```python
from build123d import *

# Parameters (mm, degrees)
F1_DEPTH = 10.4775
F2_R     = 1.5875
F3_DEPTH = 2.54
F4_R     = 0.79375
F5_DEPTH = 16.318384


with BuildPart() as f1:
    # F0 (on Front) → F1 (new body)
    with BuildSketch(Plane.XZ):
        Polygon((3.175, 15.875), (0, 15.875), (0, 0), (12.7, 0), (12.7, 4.808481), (6.430908, 5.13703), (7.012491, 16.234301), (5.427167, 16.317384), (4.7625, 3.634789), (11.1125, 3.302), (11.1125, 2.54), (3.175, 2.54), align=None)
    extrude(amount=F1_DEPTH)

    # F2 (on face) → F3 (cut)
    with BuildSketch(Plane(origin=(0, 0, 0), x_dir=(1, 0, 0), z_dir=(0, 0, -1))):
        with Locations((8.89, 5.23875)):
            Circle(F2_R)
    extrude(amount=-F3_DEPTH, mode=Mode.SUBTRACT)

    # F4 (on face) → F5 (cut, through all)
    with BuildSketch(Plane(origin=(0, 0, 0), x_dir=(1, 0, 0), z_dir=(0, 0, -1))):
        with Locations((8.89, 5.23875)):
            Circle(F4_R)
    extrude(amount=-F5_DEPTH, mode=Mode.SUBTRACT)


solid = f1.part
```
Geometry check sheet. Reference: the model listing, model coordinates, mm. A direction names the side the tool comes from. Coordinates: 2 decimals unless noted, no trailing zeros. Order: outer loops, then holes, each group sorted by start corner. A loop starts at its lowest first (then second) coordinate and runs counter-clockwise, first axis right, second up.
Item 1: Scan lines: line 1 along Y through (x, z) = (8.89, 1.8); line 2 along Y through (x, z) = (8.89, 4) (1 decimal); line 3 along Z through (x, y) = (1.5, -5.5) (3 decimals). Record each from-to range of solid material in increasing order.
Item 2: Section check C-C (z = 11.25). Enter the section's corners in (x, y) (1 decimal), plus the area to 3 significant figures.
Item 3: Tool access check on faces 4 (the flat face through (5.1, -5.2, 10.1)), 5 (the flat face through (7, -5, 2.54)), 6 (the flat face through (6.718, -5.165, 10.608)), 7 (the flat face through (2, -5, 15.875)). Record the directions out of +Z, -Z, +X, -X, +Y, -Y that give a thin tool (end or side, any length) a straight path to the whole face; none if there is none.
Item 4: Depth check by flat-ended pin: pin 1 (1 mm diameter, centred on y = -5, z = 7, fed in from +X); pin 2 (2 mm diameter, centred on y = -3, z = 10.5, fed in from +X); pin 3 (3.5 mm diameter, centred on x = 8.89, y = -5.24, fed in from +Z). Enter the tip coordinate at first touch or a pass-through.
Item 5: Section check D-D (x = 8.89). Enter the section's corners in (y, z) (1 decimal), plus the area to 3 significant figures.
Item 6: Section check B-B (y = -9.25). Enter the section's corners in (x, z) (1 decimal), plus the area to 3 significant figures.
Item 7: Section check A-A (z = 4.25). Enter the section's corners in (x, y) (1 decimal), plus the area to 3 significant figures.
Item 8: Mould release check, pull along X, two halves, no side actions. Record for faces 1 (the flat face through (6, -5, 0)), 2 (the flat face through (10.306, -5.165, 4.934)), 3 (the flat face through (7.89, -5.17, 3.47)): released by +X, released by -X, zero draft, split by the parting line, or undercut.
Check sheet entries:
1. line 1: y = -10.48 to -6.83, -3.65 to 0
1. line 2: y = -10.5 to -6, -4.4 to 0
1. line 3: z = 0 to 15.875
2. outline: (0, -10.5) - (3.2, -10.5) - (3.2, 0) - (0, 0) - close; (5.2, -10.5) - (6.8, -10.5) - (6.8, 0) - (5.2, 0) - close
2. area: 49.9 mm2
3. face 4: +Z, +Y, -Y
3. face 5: +Y, -Y
3. face 6: +X, +Y, -Y
3. face 7: +Z, -X, +Y, -Y
4. pin 1: stops at x = 6.55
4. pin 2: stops at x = 6.76
4. pin 3: stops at z = 5.1
5. outline: (-10.5, 0) - (-6.8, 0) - (-6.8, 2.5) - (-10.5, 2.5) - close; (-10.5, 3.4) - (-6, 3.4) - (-6, 5) - (-10.5, 5) - close; (-4.4, 3.4) - (0, 3.4) - (0, 5) - (-4.4, 5) - close; (-3.7, 0) - (0, 0) - (0, 2.5) - (-3.7, 2.5) - close
5. area: 32.7 mm2
6. outline: (0, 0) - (12.7, 0) - (12.7, 4.8) - (6.4, 5.1) - (7, 16.2) - (5.4, 16.3) - (4.8, 3.6) - (11.1, 3.3) - (11.1, 2.5) - (3.2, 2.5) - (3.2, 15.9) - (0, 15.9) - close
6. area: 106 mm2
7. outline: (0, -10.5) - (3.2, -10.5) - (3.2, 0) - (0, 0) - close; (4.8, -10.5) - (12.7, -10.5) - (12.7, 0) - (4.8, 0) - close; hole circle Ø1.6 at (8.9, -5.2)
7. area: 114 mm2
8. face 1: zero draft
8. face 2: released by +X
8. face 3: undercut
